Geometry: see drawing. Coordinates: mm, zero at the bounding-box minimum. A direction names the side the tool comes from. Coordinates: 2 decimals unless noted, no trailing zeros. Write each loop counter-clockwise with the first axis right and the second up, starting at its lowest first coordinate (ties: lowest second). Pieces come first, ordered by that corner, then holes.
1) Section query A-A (z = 18). Output: boundary loops of the cut face in (x, y).
2) Set-up query: the marked faces 1 and 2. Return all of +Z, -Z, +X, -X, +Y, -Y with unobstructed straight access to the full face (end or side cutting, diameter ignored); none if empty.
3) Pin query (flat end, axial travel): pin 1 Ø5 at (y, z) = (18, 18) entering from -X; pin 2 Ø10 at (y, z) = (12.5, 9.5) entering from -X; pin 3 Ø1.5 at (x, y) = (13.5, 21) entering from +Z (1 decimal); pin 4 Ø2 at (x, y) = (12, 18) entering from -Z. Return the tip coordinate at first contact, or that it passes through.
4) Line query: L1, parallel to Y at x = 17.75, z = 18; L2, parallel to Y at x = 5.75, z = 18; L3, parallel to X at y = 7.5, z = 31. Output: solid intervals per line, ascending.
5) Section query B-B (y = 18). Output: boundary loops of the cut face in (x, z), then the cut area to 3 significant figures.
6) Section query C-C (x = 10.25). Output: boundary loops of the cut face in (y, z), then the cut area to 3 significant figures.
7) Section query D-D (x = 2). Output: boundary loops of the cut face in (y, z).
8) Draft query along Y for the marked faces 3, 4 and 5. Return one class per face: pulls with the +Y half, pulls with the -Y half, needs draft (parallel to the pull), parting line crosses it, or undercut.
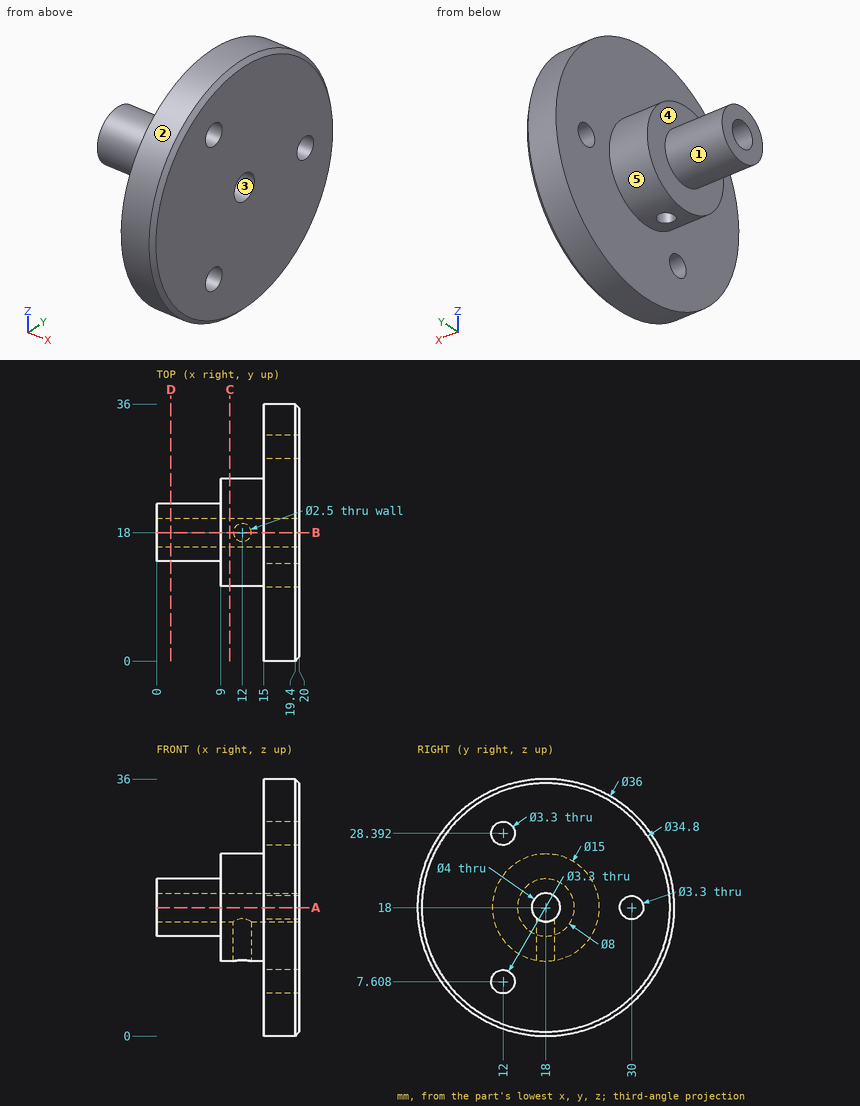
Answer:
1. outline: (0, 14) - (9, 14) - (9, 10.5) - (15, 10.5) - (15, 0) - (19.4, 0) - (20, 0.6) - (20, 16) - (0, 16) - close; (0, 20) - (20, 20) - (20, 28.35) - (15, 28.35) - (15, 25.5) - (9, 25.5) - (9, 22) - (0, 22) - close; (15, 31.65) - (20, 31.65) - (20, 35.4) - (19.4, 36) - (15, 36) - close
2. face 1: -X
2. face 2: +X, -X
3. pin 1: stops at x = 0
3. pin 2: stops at x = 9
3. pin 3: stops at z = 25.2
3. pin 4: stops at z = 19.73
4. L1: y = 0 to 16, 20 to 28.35, 31.65 to 36
4. L2: y = 14 to 16, 20 to 22
4. L3: x = 15 to 20
5. outline: (0, 14) - (9, 14) - (9, 10.5) - (10.75, 10.5) - (10.75, 16) - (0, 16) - close; (0, 20) - (20, 20) - (20, 35.4) - (19.4, 36) - (15, 36) - (15, 25.5) - (9, 25.5) - (9, 22) - (0, 22) - close; (13.25, 10.5) - (15, 10.5) - (15, 0) - (19.4, 0) - (20, 0.6) - (20, 16) - (13.25, 16) - close
5. area: 248 mm2
6. outline: circle Ø15 at (18, 18); hole circle Ø4 at (18, 18)
6. area: 164 mm2
7. outline: circle Ø8 at (18, 18); hole circle Ø4 at (18, 18)
8. face 3: undercut
8. face 4: needs draft
8. face 5: parting line crosses it
